Could you check a few things on this model? Use its own coordinates, in mm. A direction names the side the tool comes from. Round coordinates to 2 decimals unless told otherwise and drop trailing zeros. Loops run counter-clockwise (first coordinate to the right, second up) from the corner with the lowest first, then second, coordinate; pieces in that order, holes last. Notation, with made-up numbers: (-35.5, 6) -> (-2.5, 6) arc R34 ccw to (-2.5, 37) -> close; hole circle Ø2 at (73, -23). An arc over 180 degrees is marked (long way). One line per item, written item: value.
```python
from build123d import *

# Parameters (mm, degrees)
SKETCH_R        = 8
PAD_DEPTH       = 8
SKETCH001_R     = 2.4
POCKET_DEPTH    = 8.001
SKETCH002_R     = 12
SKETCH002_R_2   = 8
PAD001_DEPTH    = 35
CHAMFER_SIZE    = 0.25
CHAMFER001_SIZE = 1
CHAMFER002_SIZE = 1


with BuildPart() as housing_inner:
    # Sketch003 → Revolution (revolve)
    with BuildSketch(Plane.YZ):
        Polygon((-7.1, 6), (-7.1, 8), (-2.1, 8), (-2.1, 9), (21.1, 9), (21.1, 8), (26.1, 8), (26.1, 6), align=None)
    revolve(axis=Axis((0, 0, 0), (0, 1, 0)))


with BuildPart() as ballnut:
    # Sketch → Pad (new body)
    with BuildSketch(Plane.XZ):
        with BuildLine():
            Line((15, 15), (15, -15))
            ThreePointArc((-15, -15), (0, -21.213203), (15, -15))
            Line((-15, -15), (-15, 15))
            ThreePointArc((15, 15), (0, 21.213203), (-15, 15))
        make_face()
        Circle(SKETCH_R, mode=Mode.SUBTRACT)
    extrude(amount=PAD_DEPTH)

    # Sketch001 → Pocket (cut, through all)
    with BuildSketch(Plane.XZ.offset(8)):
        with Locations((-11.313708, 11.313708)):
            Circle(SKETCH001_R)
        with Locations((0, 16)):
            Circle(SKETCH001_R)
        with Locations((11.313708, 11.313708)):
            Circle(SKETCH001_R)
        with Locations((11.313708, -11.313708)):
            Circle(SKETCH001_R)
        with Locations((0, -16)):
            Circle(SKETCH001_R)
        with Locations((-11.313708, -11.313708)):
            Circle(SKETCH001_R)
    extrude(amount=-POCKET_DEPTH, mode=Mode.SUBTRACT)

    # Sketch002 → Pad001 (new body)
    with BuildSketch(Plane.XZ.offset(8)):
        Circle(SKETCH002_R)
        Circle(SKETCH002_R_2, mode=Mode.SUBTRACT)
    extrude(amount=-PAD001_DEPTH)

    # Chamfer
    chamfer_edges = [ballnut.edges().sort_by_distance(p)[0] for p in [
        (0, -8, 21.213203),
        (0, 0, 21.213203),
        (15, 0, 0),
        (15, -8, 0),
        (0, 0, -21.213203),
        (0, -8, -21.213203),
        (-15, -8, 0),
        (-15, 0, 0),
    ]]
    chamfer(chamfer_edges, length=CHAMFER_SIZE)

    # Chamfer001
    chamfer001_edges = [ballnut.edges().sort_by_distance(p)[0] for p in [
        (-8, -8, 0),
    ]]
    chamfer(chamfer001_edges, length=CHAMFER001_SIZE)

    # Chamfer002
    chamfer002_edges = [ballnut.edges().sort_by_distance(p)[0] for p in [
        (-8, 27, 0),
    ]]
    chamfer(chamfer002_edges, length=CHAMFER002_SIZE)

    # Fusion: union housing-inner
    add(housing_inner.part)


solid = ballnut.part
```
(1) Imagine slicing it at A-A on z = 0. Write out the boundary of the cut face in (x, y), then the cut area to 3 significant figures.
Results below:
outline: (-15, -7.75) -> (-14.75, -8) -> (-9, -8) -> (-8, -7) -> (-8, -7.1) -> (-6, -7.1) -> (-6, 26.1) -> (-8, 26.1) -> (-8, 26) -> (-9, 27) -> (-12, 27) -> (-12, 0) -> (-14.75, 0) -> (-15, -0.25) -> close; (6, -7.1) -> (8, -7.1) -> (8, -7) -> (9, -8) -> (14.75, -8) -> (15, -7.75) -> (15, -0.25) -> (14.75, 0) -> (12, 0) -> (12, 27) -> (9, 27) -> (8, 26) -> (8, 26.1) -> (6, 26.1) -> close
area: 459 mm²
(2) Imagine slicing it at B-B on y = 2. Write out the boundary of the cut face in (x, z).
Results below:
outline: circle Ø24 at (0, 0); hole circle Ø12 at (0, 0)
(3) On a 3-axis mill with a long thin cutter (end or side, diameter ignored), from which of +Z, -Z, +X, -X, +Y, -Y can I reach the whole of each face in a straight line? I mean faces 4 (the face through (10, 0, -9)), 5 (the face through (9.545, -4.056, -9.692)), 6 (the face through (6, -7.1, 2)). Say none if no direction works.
Results below:
face 4: +Y
face 5: +Y, -Y
face 6: -Y
(4) For pin 1 Ø5 at (x, z) = (-2.5, 4) entering from +Y; pin 2 Ø5.5 at (x, z) = (11.31, -11.31) entering from +Y; pin 3 Ø8 at (x, y) = (1, 14.5) entering from -Z, each with a flat end and sliding along its axis, tell me the tip position at first contact or that it passes through.
Results below:
pin 1: stops at y = 26.1
pin 2: stops at y = 0
pin 3: stops at z = -12
(5) Please list where these lines run through material, in increasing order: L1, parallel to Z at x = -11.5, y = -2.5; L2, parallel to X at y = -2, z = 10.5; L3, parallel to Y at x = 9, z = 14.
Results below:
L1: z = -17.83 to -13.71, -8.92 to 8.92, 13.71 to 17.83
L2: x = -15 to -13.57, -9.06 to 9.06, 13.57 to 15
L3: y = -8 to 0
(6) Imagine slicing it at C-C on x = 0. Give the number of separate pieces and of enclosed holes in the cut face, then the cut area to 3 significant figures.
Results below:
separate pieces: 4
enclosed holes: 0
area: 481 mm²
(7) We'd pull the mould along Z, two halves only. Please class faces 1 (the face through (1.29, -4.056, -13.976)), 2 (the face through (-0.23, -3.95, -21.21)), 3 (the face through (0.23, -3.95, 21.21)): +Z half, -Z half, draft (parallel to the pull), parting line (faces both ways), or undercut.
Results below:
face 1: undercut
face 2: -Z half
face 3: +Z half
